Answer from the drawing. Dimensions are ordinates in mm from the lowest x, y and z of the part. A direction names the side the tool comes from. Coordinates: 2 decimals unless noted, no trailing zeros. Order: outer loops, then holes, each group sorted by start corner. A loop starts at its lowest first (then second) coordinate and runs counter-clockwise, first axis right, second up. Notation, with made-up numbers: M 43.25,7 L 92.25,7 A14 ccw 92.25,30 Z; hole C 33,26.25 d5. An arc over 180 degrees is marked long. Use a Markdown table: item, result.
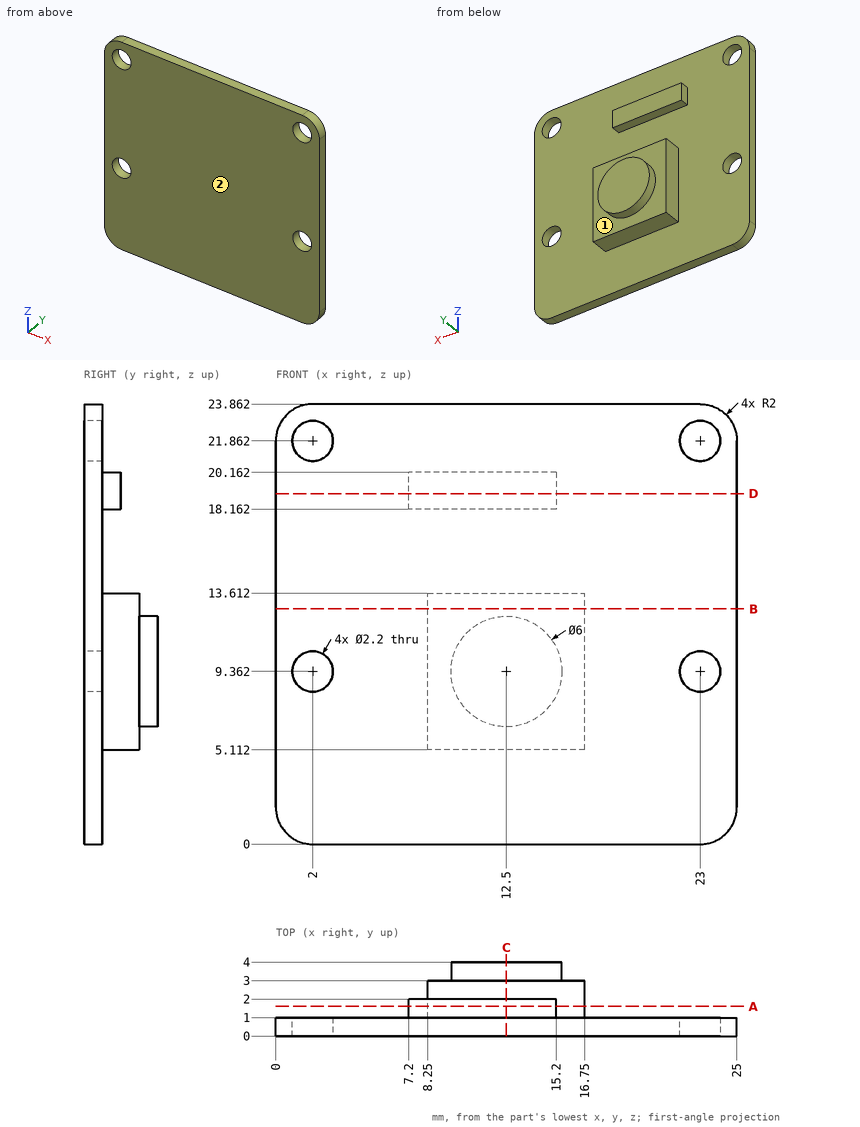
(1) Straight lines are drawn through the part: L1, parallel to Z at x = 23, y = 0.4; L2, parallel to Z at x = 9.75, y = 1.25; L3, parallel to X at y = 0.85, z = 8.5. For each, find the intervals that lie inside material, in ascending order.
Conclusion:
| item | result |
|---|---|
| L1 | 0 to 8.26, 10.46 to 20.76, 22.96 to 23.86 |
| L2 | 5.11 to 13.61, 18.16 to 20.16 |
| L3 | 0 to 1.32, 2.68 to 22.32, 23.68 to 25 |
(2) A cutting plane is placed at C-C (x = 12.5). Determine the outline of the cut face in (y, z), then the cut area to 3 significant figures.
Conclusion:
| item | result |
|---|---|
| outline | M 0,0 L 1,0 L 1,5.11 L 3,5.11 L 3,6.36 L 4,6.36 L 4,12.36 L 3,12.36 L 3,13.61 L 1,13.61 L 1,18.16 L 2,18.16 L 2,20.16 L 1,20.16 L 1,23.86 L 0,23.86 Z |
| area | 48.9 mm2 |
(3) A cutting plane is placed at A-A (y = 1.6). Determine the outline of the cut face in (x, z).
Conclusion:
| item | result |
|---|---|
| outline | M 7.2,18.16 L 15.2,18.16 L 15.2,20.16 L 7.2,20.16 Z; M 8.25,5.11 L 16.75,5.11 L 16.75,13.61 L 8.25,13.61 Z |
(4) A cutting plane is placed at D-D (z = 19). Determine the outline of the cut face in (x, y), then the cut area to 3 significant figures.
Conclusion:
| item | result |
|---|---|
| outline | M 0,0 L 25,0 L 25,1 L 15.2,1 L 15.2,2 L 7.2,2 L 7.2,1 L 0,1 Z |
| area | 33.0 mm2 |
(5) Given P1, Ø12, axis at x = 12.5, z = 15.5, coming from the +Y side; P2, Ø0.6, axis at x = 11.5, y = 2, coming from the +Z side; P3, Ø0.8, axis at x = 11, y = 1.5, coming from the -Z side; P4, Ø2, axis at x = 10, z = 19, coming from the +Y side, each flat-ended and moving along its own axis, determine where each tip first touches the part or whether it passes through.
Conclusion:
| item | result |
|---|---|
| P1 | y = 4 |
| P2 | z = 20.16 |
| P3 | z = 5.11 |
| P4 | y = 2 |
(6) A cutting plane is placed at B-B (z = 12.75). Determine the outline of the cut face in (x, y), then the cut area to 3 significant figures.
Conclusion:
| item | result |
|---|---|
| outline | M 0,0 L 25,0 L 25,1 L 16.75,1 L 16.75,3 L 8.25,3 L 8.25,1 L 0,1 Z |
| area | 42.0 mm2 |
(7) Which of the six approach directions +Z, -Z, +X, -X, +Y, -Y give full straight-line access (tool end or side, diameter ignored) to the marked faces 1 and 2?
Conclusion:
| item | result |
|---|---|
| face 1 | +Y |
| face 2 | +Z, -Z, +X, -X, -Y |
